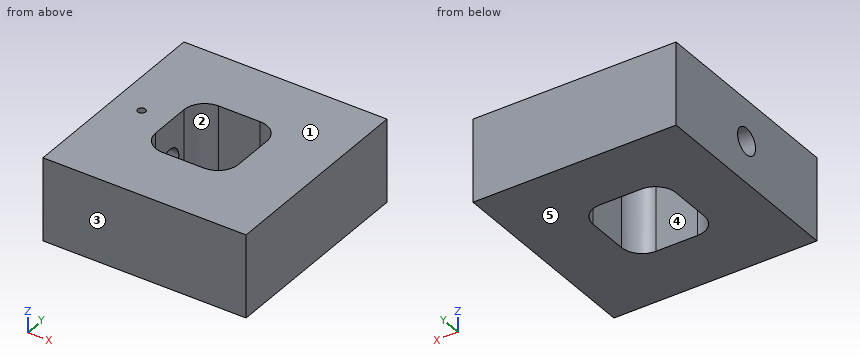
from build123d import *

# Parameters (mm, degrees)
F0_W     = 62.23
F0_H     = 63.5
F1_DEPTH = 25.4
F3_D     = 8.1026
F3_DEPTH = 20.32
F5_D     = 2.3876
F5_DEPTH = 12.7


with BuildPart() as f1:
    # F0 (on Top) → F1 (new body)
    with BuildSketch(Plane.XY):
        with Locations((1.843547, 12.7)):
            Rectangle(F0_W, F0_H)
        with BuildLine():
            ThreePointArc((-11.999453, 19.05), (-10.139581, 23.540128), (-5.649453, 25.4))
            Line((-5.649453, 25.4), (7.050547, 25.4))
            ThreePointArc((7.050547, 25.4), (11.540676, 23.540128), (13.400547, 19.05))
            Line((13.400547, 19.05), (13.400547, 6.35))
            ThreePointArc((13.400547, 6.35), (11.540676, 1.859872), (7.050547, 0))
            Line((7.050547, 0), (-5.649453, 0))
            ThreePointArc((-5.649453, 0), (-10.139581, 1.859872), (-11.999453, 6.35))
            Line((-11.999453, 6.35), (-11.999453, 19.05))
        make_face(mode=Mode.SUBTRACT)
    extrude(amount=F1_DEPTH)

    # F3
    with Locations(Plane(origin=(-29.271453, 0, 0), x_dir=(0, -1, 0), z_dir=(-1, 0, 0))):
        with Locations((-12.7, 12.7)):
            Hole(F3_D / 2, depth=F3_DEPTH)

    # F5
    with Locations(Plane.XY.offset(25.4)):
        with Locations((-20.635453, 12.7)):
            Hole(F5_D / 2, depth=F5_DEPTH)


solid = f1.part
Part model, mm, in its own coordinate system. Face numbers are marked on the shaded views. A direction names the side the tool comes from. Give positions to 0.01 mm unless a question says otherwise; leave off trailing zeros. Loops run counter-clockwise (first coordinate to the right, second up) from the corner with the lowest first, then second, coordinate; pieces in that order, holes last. Notation, with made-up numbers: M 42.5,21 L 87.5,21 A14 cw 87.5,48 Z; hole C -24,49 d1. An arc over 180 degrees is marked long. Put each result on its own line as item: value. Start each with the question number.
1) Probe probe 1 along X at (y, z) = (12.7, 23); probe 2 along Z at (x, y) = (-16.75, 12.7); probe 3 along Y at (x, z) = (7.5, 19.5). List the from-to ranges inside material, lowest first.
2) Saw through at C-C (z = 21.25). List the corners of the cut face in (x, y), then the cut area to 3 significant figures.
3) Pull direction Y, two halves, no side cores. Call the marked faces 1, 2 and 3: +Y half, -Y half, draft (parallel to the pull), parting line (faces both ways), or undercut.
4) Saw through at B-B (x = -2). List the corners of the cut face in (y, z), then the cut area to 3 significant figures.
5) 3-axis set-ups, long thin cutter, end or side, ignore diameter. For the marked faces 4 and 5: which of +Z, -Z, +X, -X, +Y, -Y reach the whole face in a straight line?
6) Saw through at D-D (x = -18). List the corners of the cut face in (y, z), then the cut area to 3 significant figures.
7) Saw through at A-A (y = 12.7). List the corners of the cut face in (x, z), then the cut area to 3 significant figures.
Numbers:
1. probe 1: -29.27 to -21.83, -19.44 to -12, 13.4 to 32.96
1. probe 2: 0 to 8.65, 16.75 to 25.4
1. probe 3: -19.05 to 0.02, 25.38 to 44.45
2. outline: M -29.27,-19.05 L 32.96,-19.05 L 32.96,44.45 L -29.27,44.45 Z; hole C -20.64,12.7 d2.39; hole M -12,6.35 A6.35 ccw -5.65,0 L 7.05,0 A6.35 ccw 13.4,6.35 L 13.4,19.05 A6.35 ccw 7.05,25.4 L -5.65,25.4 A6.35 ccw -12,19.05 Z
2. area: 3,340 mm^2
3. face 1: draft
3. face 2: undercut
3. face 3: -Y half
4. outline: M -19.05,0 L 0,0 L 0,25.4 L -19.05,25.4 Z; M 25.4,0 L 44.45,0 L 44.45,25.4 L 25.4,25.4 Z
4. area: 968 mm^2
5. face 4: +Z, -Z
5. face 5: -Z, +X, -X, +Y, -Y
6. outline: M -19.05,0 L 44.45,0 L 44.45,25.4 L -19.05,25.4 Z; hole C 12.7,12.7 d8.1
6. area: 1,560 mm^2
7. outline: M -29.27,0 L -12,0 L -12,8.65 L -29.27,8.65 Z; M -29.27,16.75 L -21.83,16.75 L -21.83,25.4 L -29.27,25.4 Z; M -19.44,16.75 L -12,16.75 L -12,25.4 L -19.44,25.4 Z; M 13.4,0 L 32.96,0 L 32.96,25.4 L 13.4,25.4 Z
7. area: 775 mm^2
